The model under review builds one solid part; all positions refer to its coordinate system, in mm. Face numbers are marked on the shaded views. A direction names the side the tool comes from. Round coordinates to 2 decimals unless told otherwise and drop trailing zeros. Write each loop counter-clockwise with the first axis right and the second up, starting at its lowest first coordinate (ties: lowest second). Pieces come first, ordered by that corner, then holes. Notation, with made-up numbers: (33.25, 27.25) -> (47.25, 27.25) arc R10 ccw to (47.25, 38.25) -> close; hole circle Ø3 at (85, -38). An arc over 180 degrees is marked (long way). Return JSON: item names as keys, results as strings. Group by question number.
1. For line 1 along Z through (x, y) = (0, -47.5); line 2 along X through (y, z) = (-6.5, -1); line 3 along Y through (x, z) = (3, -1.75), list the stretches that pass through material, from the lowest coordinate up. Write a range as from..to.
2. Take a section at A-A, the plane y = -8. Write out the cut boundary in (x, z), then the cut area to 3 significant figures.
3. Tool access review of the marked faces 4 and 5: name each direction out of +Z, -Z, +X, -X, +Y, -Y from which nothing blocks a thin tool from reaching the whole face with its end or side.
4. Mouldability with a two-part tool opening along Z and no side actions: class the marked faces 1, 2 and 3 as pulls with the +Z half, pulls with the -Z half, needs draft (parallel to the pull), parting line crosses it, or undercut.
5. Clearance check with flat-ended pins moving along their axes: P1, Ø5, axis at x = -2, y = -15.5, coming from the +Z side; P2, Ø2, axis at y = -39.5, z = -4, coming from the +X side; P3, Ø1, axis at y = -27, z = 5.5, coming from the +X side; P4, Ø4, axis at x = 5.5, y = -11.5, coming from the +Z side. State where each tip first meets the part, or that it passes through.
6. Take a section at B-B, the plane y = -46. Write out the cut boundary in (x, z).
from build123d import *

# Parameters (mm, degrees)
F1_DEPTH = 12
F2_R     = 4.25
F2_R_2   = 3.5
F3_DEPTH = 50
F4_R     = 1.27


with BuildPart() as f1:
    # F0 (on Front) → F1 (new body)
    with BuildSketch(Plane.XZ):
        Polygon((0.015132, -8.660241), (7.507554, -4.317016), (7.492423, 4.343225), (-0.015132, 8.660241), (-7.507554, 4.317016), (-7.492423, -4.343225), align=None)
    extrude(amount=F1_DEPTH)

    # F2 (on face) → F3 (join)
    with BuildSketch(Plane.XZ.offset(12)):
        Circle(F2_R)
        Circle(F2_R_2, mode=Mode.SUBTRACT)
    extrude(amount=F3_DEPTH)

    # F4
    f4_edges = [f1.edges().sort_by_distance(p)[0] for p in [
        (7.492423, -6, 4.343225),
        (-0.015132, -6, 8.660241),
        (3.738645, 0, 6.501733),
        (3.738645, -12, 6.501733),
        (7.507554, -6, -4.317016),
        (7.499989, 0, 0.013105),
        (7.499989, -12, 0.013105),
        (-7.507554, -6, 4.317016),
        (-3.761343, 0, 6.488628),
        (-3.761343, -12, 6.488628),
        (-7.492423, -6, -4.343225),
        (-7.499989, 0, -0.013105),
        (-7.499989, -12, -0.013105),
        (0.015132, -6, -8.660241),
        (-3.738645, 0, -6.501733),
        (-3.738645, -12, -6.501733),
        (3.761343, 0, -6.488628),
        (3.761343, -12, -6.488628),
    ]]
    fillet(f4_edges, radius=F4_R)


solid = f1.part
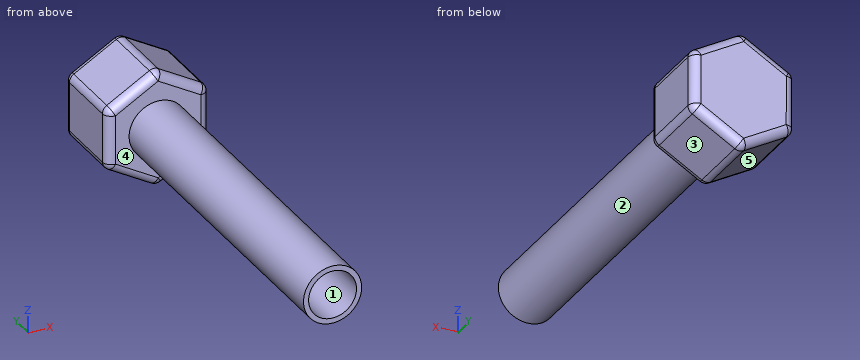
Output:
{
 "1": {"line 1": "z = -4.25..-3.5, 3.5..4.25", "line 2": "x = -7.5..7.5", "line 3": "y = -12..0"},
 "2": {"outline": "(-7.51, 3.58) -> (-7.49, -3.61) arc R1.27 ccw to (-6.86, -4.71) -> (-0.62, -8.29) arc R1.27 ccw to (0.65, -8.29) -> (6.87, -4.68) arc R1.27 ccw to (7.51, -3.58) -> (7.49, 3.61) arc R1.27 ccw to (6.86, 4.71) -> (0.62, 8.29) arc R1.27 ccw to (-0.65, 8.29) -> (-6.87, 4.68) arc R1.27 ccw to start", "area": "194 mm^2"},
 "3": {"face 4": "-Y", "face 5": "-Z, -X, +Y, -Y"},
 "4": {"face 1": "undercut", "face 2": "parting line crosses it", "face 3": "pulls with the -Z half"},
 "5": {"P1": "stops at z = 4.25", "P2": "stops at x = 3.01", "P3": "passes through", "P4": "stops at z = 6.57"},
 "6": {"outline": "circle Ø8.5 at (0, 0); hole circle Ø7 at (0, 0)"}
}
